```python
from build123d import *

# Parameters (mm, degrees)
SKETCH_1_W             = 12
SKETCH_1_H             = 23
EXTRUDE_1_DEPTH        = 10
SKETCH_3_W             = 12
SKETCH_3_H             = 3
CUT_EXTRUDE_1_DEPTH    = 4.5
SKETCH_4_W             = 1
SKETCH_4_H             = 3
CUT_EXTRUDE_2_DEPTH    = 11
CUT_EXTRUDE_3_DEPTH    = 6
CUT_EXTRUDE_4_DEPTH    = 1
FILLET_1_R             = 1.5
FILLET_2_R             = 2
FILLET_1_OF_MIRROR_1_R = 1.5
FILLET_2_OF_MIRROR_1_R = 2
SKETCH_7_W             = 6
SKETCH_7_H             = 11.5
CUT_EXTRUDE_5_DEPTH    = 4
SKETCH_8_W             = 8
SKETCH_8_H             = 16
CUT_EXTRUDE_6_DEPTH    = 8
SKETCH_9_R             = 2.5
CUT_EXTRUDE_7_DEPTH    = 4
EXTRUDE_2_DEPTH        = 2
SKETCH_11_R            = 1.25
CUT_EXTRUDE_8_DEPTH    = 5
CUT_EXTRUDE_9_DEPTH    = 2
CHAMFER_1_SIZE         = 0.3
SKETCH_13_R            = 1.25
EXTRUDE_3_DEPTH        = 15
FILLET_3_R             = 1.25


with BuildPart() as part:
    # 草图1 → 凸台-拉伸1 (new body)
    with BuildSketch(Plane(origin=(0, 0, 0), x_dir=(1, 0, 0), z_dir=(0, 1, 0))):
        Rectangle(SKETCH_1_W, SKETCH_1_H)
    extrude(amount=EXTRUDE_1_DEPTH)

    # 草图3 → 切除-拉伸1 (cut)
    with BuildSketch(Plane(origin=(0, 10, 0), x_dir=(1, 0, 0), z_dir=(0, 1, 0))):
        with Locations((0, -10)):
            Rectangle(SKETCH_3_W, SKETCH_3_H)
    extrude(amount=-CUT_EXTRUDE_1_DEPTH, mode=Mode.SUBTRACT)

    # 草图4 → 切除-拉伸2 (cut, through all)
    with BuildSketch(Plane(origin=(0, 0, 0), x_dir=(1, 0, 0), z_dir=(0, 1, 0))):
        with Locations((5.5, -10)):
            Rectangle(SKETCH_4_W, SKETCH_4_H)
        with Locations((-5.5, -10)):
            Rectangle(SKETCH_4_W, SKETCH_4_H)
    extrude(amount=CUT_EXTRUDE_2_DEPTH, mode=Mode.SUBTRACT)

    # 草图5 → 切除-拉伸3 (cut, symmetric)
    with BuildSketch(Plane(origin=(0, 0, 0), x_dir=(0, 0, -1), z_dir=(1, 0, 0))):
        with BuildLine():
            Line((11.5, 5.5), (0, 5.5))
            ThreePointArc((0, 5.5), (-4.042500986, 3.686592074), (-6.5, 0))
            Line((-6.5, 0), (11.5, 0))
            Line((11.5, 0), (11.5, 5.5))
        make_face()
        Polygon((-9, 0), (-11.5, 4), (-11.5, 0), align=None)
    extrude(amount=CUT_EXTRUDE_3_DEPTH, both=True, mode=Mode.SUBTRACT)

    # 草图6 → 切除-拉伸4 (cut)
    with BuildSketch(Plane(origin=(6, 0, 0), x_dir=(0, 0, -1), z_dir=(1, 0, 0))):
        with BuildLine():
            Line((-8.5, 4), (-4.5, 4))
            Line((-4.5, 4), (-3, 5.5))
            Line((-3, 5.5), (0, 5.5))
            ThreePointArc((0, 5.5), (-4.042500986, 3.686592074), (-6.5, 0))
            Line((-6.5, 0), (-8.5, 0))
            Line((-8.5, 0), (-8.5, 4))
        make_face()
    cut_extrude_4 = extrude(amount=-CUT_EXTRUDE_4_DEPTH, mode=Mode.SUBTRACT)

    # 圆角1
    fillet_1_edges = [part.edges().sort_by_distance(p)[0] for p in [
        (5.5, 4, 4.5),
    ]]
    fillet(fillet_1_edges, radius=FILLET_1_R)

    # 圆角2
    fillet_2_edges = [part.edges().sort_by_distance(p)[0] for p in [
        (5.5, 5.5, 3),
    ]]
    fillet(fillet_2_edges, radius=FILLET_2_R)

    # 镜向1: 切除-拉伸4 across plane
    add(cut_extrude_4.mirror(Plane(origin=(0, 0, 0), x_dir=(0, 0, 1), z_dir=(1, 0, 0))), mode=Mode.SUBTRACT)

    # 圆角1 of 镜向1
    fillet_1_of_mirror_1_edges = [part.edges().sort_by_distance(p)[0] for p in [
        (-5.5, 4, 4.5),
    ]]
    fillet(fillet_1_of_mirror_1_edges, radius=FILLET_1_OF_MIRROR_1_R)

    # 圆角2 of 镜向1
    fillet_2_of_mirror_1_edges = [part.edges().sort_by_distance(p)[0] for p in [
        (-5.5, 5.5, 3),
    ]]
    fillet(fillet_2_of_mirror_1_edges, radius=FILLET_2_OF_MIRROR_1_R)

    # 草图7 → 切除-拉伸5 (cut)
    with BuildSketch(Plane(origin=(0, 0, 0), x_dir=(1, 0, 0), z_dir=(0, 1, 0))):
        with Locations((0, -5.75)):
            Rectangle(SKETCH_7_W, SKETCH_7_H)
    extrude(amount=CUT_EXTRUDE_5_DEPTH, mode=Mode.SUBTRACT)

    # 草图8 → 切除-拉伸6 (cut)
    with BuildSketch(Plane(origin=(0, 0, 0), x_dir=(1, 0, 0), z_dir=(0, 1, 0))):
        with Locations((0, 1.5)):
            Rectangle(SKETCH_8_W, SKETCH_8_H)
    extrude(amount=CUT_EXTRUDE_6_DEPTH, mode=Mode.SUBTRACT)

    # 草图9 → 切除-拉伸7 (cut)
    with BuildSketch(Plane.XZ.offset(-4)):
        with Locations((0, 4.5)):
            Circle(SKETCH_9_R)
    extrude(amount=-CUT_EXTRUDE_7_DEPTH, mode=Mode.SUBTRACT)

    # 草图10 → 凸台-拉伸2 (add)
    with BuildSketch(Plane.XZ.offset(-8)):
        with BuildLine():
            Line((2, 1), (3, 2))
            Line((3, 2), (3, 6.5))
            Line((3, 6.5), (1.5, 6.5))
            ThreePointArc((1.5, 6.5), (0, 7), (-1.5, 6.5))
            Line((-1.5, 6.5), (-3, 6.5))
            Line((-3, 6.5), (-3, 2))
            Line((-3, 2), (-2, 1))
            Line((-2, 1), (-2, -0.5))
            Line((-2, -0.5), (2, -0.5))
            Line((2, -0.5), (2, 1))
        make_face()
    extrude(amount=EXTRUDE_2_DEPTH)

    # 草图11 → 切除-拉伸8 (cut, through all)
    with BuildSketch(Plane.XZ.offset(-6)):
        with Locations((0, 4.5)):
            Circle(SKETCH_11_R)
    extrude(amount=-CUT_EXTRUDE_8_DEPTH, mode=Mode.SUBTRACT)

    # 草图12 → 切除-拉伸9 (cut)
    with BuildSketch(Plane(origin=(0, 10, 0), x_dir=(1, 0, 0), z_dir=(0, 1, 0))):
        with BuildLine():
            Line((-0.75, -1.25), (0.75, -1.25))
            Line((0.75, -1.25), (0.75, -2.115151996))
            ThreePointArc((0.75, -2.115151996), (2.5, -4.5), (0.75, -6.884848004))
            Line((0.75, -6.884848004), (0.75, -7.75))
            Line((0.75, -7.75), (-0.75, -7.75))
            Line((-0.75, -7.75), (-0.75, -6.884848004))
            ThreePointArc((-0.75, -6.884848004), (-2.5, -4.5), (-0.75, -2.115151996))
            Line((-0.75, -2.115151996), (-0.75, -1.25))
        make_face()
    extrude(amount=-CUT_EXTRUDE_9_DEPTH, mode=Mode.SUBTRACT)

    # 倒角1
    chamfer_1_edges = [part.edges().sort_by_distance(p)[0] for p in [
        (2.5, 10, 4.5),
        (0.75, 10, 1.682575998),
        (0, 10, 1.25),
        (-0.75, 10, 1.682575998),
        (-2.5, 10, 4.5),
        (-0.75, 10, 7.317424002),
        (0, 10, 7.75),
        (0.75, 10, 7.317424002),
    ]]
    chamfer(chamfer_1_edges, length=CHAMFER_1_SIZE)

    # 草图13 → 凸台-拉伸3 (add)
    with BuildSketch(Plane(origin=(0, 0, -11.5), x_dir=(-1, 0, 0), z_dir=(0, 0, -1))):
        with Locations((0, 8.5)):
            Circle(SKETCH_13_R)
    extrude(amount=EXTRUDE_3_DEPTH)

    # 圆角3
    fillet_3_edges = [part.edges().sort_by_distance(p)[0] for p in [
        (1.25, 8.5, -26.5),
    ]]
    fillet(fillet_3_edges, radius=FILLET_3_R)


solid = part.part
```
Design review of the part built by this model. Coordinates are the model's own, in mm. A direction names the side the tool comes from. Round coordinates to 2 decimals unless told otherwise and drop trailing zeros. Write each loop counter-clockwise with the first axis right and the second up, starting at its lowest first coordinate (ties: lowest second). Pieces come first, ordered by that corner, then holes. Notation, with made-up numbers: (23.25, -2) -> (57.25, -2) arc R21 cw to (57.25, 13) -> close; hole circle Ø11 at (-22, 86). An arc over 180 degrees is marked (long way). Write item = value, one per line. Start each with the question number.
1) Take a section at A-A, the plane x = 0. State the section outline as (y, z) points, plus the area to 3 significant figures.
2) Take a section at C-C, the plane y = 1. State the section outline as (x, z) points (3 decimals).
3) Wall thickness on probe 1 along Z at (x, y) = (0, 6.75); probe 2 along Z at (x, y) = (-1.5, 6.25); probe 3 along Z at (x, y) = (2.25, 7.5): over which ranges is each line inside the solid? List them lowest first. Write a range as from..to.
4) Take a section at D-D, the plane y = 8.5. State the section outline as (x, z) points, plus the area to 3 significant figures.
5) Clearance check with flat-ended pins moving along their axes: pin 1 (1.2 mm diameter, centred on x = -0.5, y = 9, fed in from -Z); pin 2 (1.2 mm diameter, centred on x = 1.5, y = 6.5, fed in from +Z); pin 3 (3.5 mm diameter, centred on x = 2.5, y = 8.5, fed in from -Z). State where each tip first meets the part, or that it passes through.
6) Tool access review of faces 3 (the face through (-5.493, 5.344, 2.947)), 4 (the face through (-0.27, 6.99, 3.28)), 5 (the face through (-2.62, 9.82, 4.55)), 6 (the face through (1, 6, 3)), 7 (the face through (4.01, 1.97, 10.23)): name each direction out of +Z, -Z, +X, -X, +Y, -Y from which nothing blocks a thin tool from reaching the whole face with its end or side.
7) Take a section at B-B, the plane z = 4.5. State the section outline as (x, y) points, plus the area to 3 significant figures.
8) Mouldability with a two-part tool opening along X and no side actions: class faces 1 (the face through (0, 5.5, 10)), 2 (the face through (2.5, 8.9, 4.5)) as +X half, -X half, draft (parallel to the pull), parting line (faces both ways), or undercut.
Results list:
q1.outline = (4, 7) -> (6, 7) -> (6, 5.75) -> (8, 5.75) -> (8, 7.75) -> (9.7, 7.75) -> (10, 8.05) -> (10, 8.5) -> (5.5, 8.5) -> (5.5, 11.5) -> (4, 11.5) -> close; (5.5, -11.5) -> (7.25, -11.5) -> (7.25, -25.25) arc R1.25 ccw to (9.75, -25.25) -> (9.75, -11.5) -> (10, -11.5) -> (10, 0.95) -> (9.7, 1.25) -> (8, 1.25) -> (8, 3.25) -> (6, 3.25) -> (6, -0.5) -> (8, -0.5) -> (8, -9.5) -> (5.5, -9.5) -> close
q1.area = 89.2 mm²
q2.outline = (-5, 6.107) -> (-4, 6.107) -> (-4, 6.5) -> (-3, 6.5) -> (-3, 9.625) -> (-5, 9.625) -> close; (3, 6.5) -> (4, 6.5) -> (4, 6.107) -> (5, 6.107) -> (5, 9.625) -> (3, 9.625) -> close
q3.probe_1 = -11.5..-9.5, -0.5..3.25, 5.75..8.5
q3.probe_2 = -11.5..-9.5, -0.5..8.5
q3.probe_3 = -11.5..-9.5, 1.25..8.5
q4.outline = (-6, -11.5) -> (-1.25, -11.5) -> (-1.25, -25.25) arc R1.25 ccw to (1.25, -25.25) -> (1.25, -11.5) -> (6, -11.5) -> (6, 8.5) -> (-6, 8.5) -> close; hole (-0.75, 1.25) -> (0.75, 1.25) -> (0.75, 2.12) arc R2.5 ccw to (0.75, 6.88) -> (0.75, 7.75) -> (-0.75, 7.75) -> (-0.75, 6.88) arc R2.5 ccw to (-0.75, 2.12) -> close
q4.area = 255 mm²
q5.pin_1 = -26.5
q5.pin_2 = 8.5
q5.pin_3 = -26.25
q6.face_3 = -Z, -X, -Y
q6.face_4 = +Y, -Y
q6.face_5 = +Y
q6.face_6 = -Y
q6.face_7 = +Z, +X, -X, -Y
q7.outline = (-6, 4.13) -> (-5, 4.13) -> (-5, 3.27) -> (-4, 3.27) -> (-4, 8) -> (-3, 8) -> (-3, 6) -> (-1.25, 6) -> (-1.25, 8) -> (-2.5, 8) -> (-2.5, 9.7) -> (-2.8, 10) -> (-6, 10) -> close; (1.25, 6) -> (3, 6) -> (3, 8) -> (4, 8) -> (4, 3.27) -> (5, 3.27) -> (5, 4.13) -> (6, 4.13) -> (6, 10) -> (2.8, 10) -> (2.5, 9.7) -> (2.5, 8) -> (1.25, 8) -> close
q7.area = 38.1 mm²
q8.face_1 = draft
q8.face_2 = undercut
